Model file for the job. Use its own axes, mm. Face numbers are marked on the shaded views. A direction names the side the tool comes from. Round coordinates to 2 decimals unless told otherwise and drop trailing zeros. Loops run counter-clockwise (first coordinate to the right, second up) from the corner with the lowest first, then second, coordinate; pieces in that order, holes last. Notation, with made-up numbers: (48.5, 1.25) -> (100.5, 1.25) arc R5 cw to (100.5, 5.25) -> close; hole circle Ø10 at (22.5, -8.5). An arc over 180 degrees is marked (long way). Use a Markdown table: item, result.
from build123d import *

# Parameters (mm, degrees)
SKETCH2_R           = 0.6
BOSS_EXTRUDE2_DEPTH = 5
BOSS_EXTRUDE4_START = 15
BOSS_EXTRUDE4_DEPTH = 15
SKETCH8_R           = 1.5
CUT_EXTRUDE2_DEPTH  = 21.756494148


with BuildPart() as part:
    # Sketch2 → Boss-Extrude2 (new body)
    with BuildSketch(Plane.XY):
        with BuildLine():
            Line((-11.842719282, 4), (11.842719282, 4))
            Line((11.842719282, 4), (12.369316877, 4))
            ThreePointArc((12.369316877, 4), (13, 0), (12.369316877, -4))
            Line((12.369316877, -4), (11.842719282, -4))
            Line((11.842719282, -4), (-11.842719282, -4))
            Line((-11.842719282, -4), (-12.369316877, -4))
            ThreePointArc((-12.369316877, -4), (-13, 0), (-12.369316877, 4))
            Line((-12.369316877, 4), (-11.842719282, 4))
        make_face()
        with Locations((10, 0)):
            Circle(SKETCH2_R, mode=Mode.SUBTRACT)
        with Locations(Location((-10, 0, 0), (0, 0, 180))):
            Circle(SKETCH2_R, mode=Mode.SUBTRACT)
    extrude(amount=BOSS_EXTRUDE2_DEPTH)

    # Sketch7 → Boss-Extrude4 (add)
    with BuildSketch(Plane(origin=(0, 0, 0), x_dir=(-1, 0, 0), z_dir=(0, 0, -1)).offset(BOSS_EXTRUDE4_START)):
        with BuildLine():
            Line((0, -2.068941366), (-12.32759026, -2.068941366))
            Line((-12.32759026, -2.068941366), (-12.834308771, -2.068941366))
            ThreePointArc((-12.834308771, -2.068941366), (-12.6387473, -3.04336437), (-12.369316877, -4))
            Line((-12.369316877, -4), (-11.842719282, -4))
            Line((-11.842719282, -4), (0, -4))
            Line((0, -4), (11.842719282, -4))
            Line((11.842719282, -4), (12.369316877, -4))
            ThreePointArc((12.369316877, -4), (12.6387473, -3.04336437), (12.834308771, -2.068941366))
            Line((12.834308771, -2.068941366), (12.32759026, -2.068941366))
            Line((12.32759026, -2.068941366), (0, -2.068941366))
        make_face()
    extrude(amount=-BOSS_EXTRUDE4_DEPTH)

    # Sketch8 → Cut-Extrude2 (cut, through all)
    with BuildSketch(Plane(origin=(0, -2.068941366, 0), x_dir=(1, 0, 0), z_dir=(0, 1, 0))):
        with Locations(Location((-10.795, 7.5, 0), (0, 0, 270))):
            Circle(SKETCH8_R)
        with Locations(Location((10.795, 7.5, 0), (0, 0, 90))):
            Circle(SKETCH8_R)
    extrude(amount=-CUT_EXTRUDE2_DEPTH, mode=Mode.SUBTRACT)


solid = part.part
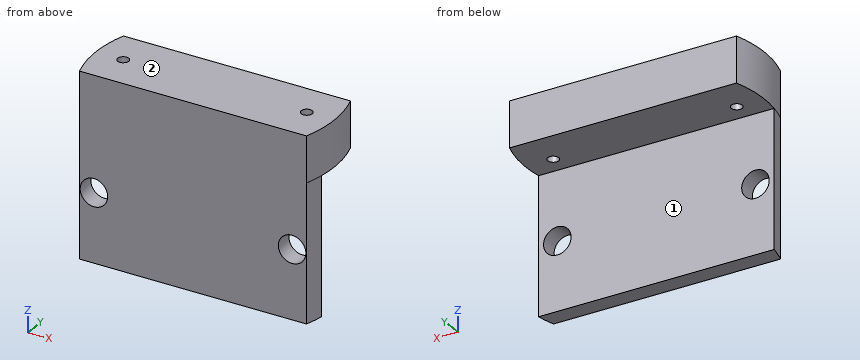
Q1. Flat gauge pins, fed straight in: pin 1 (10 mm diameter, centred on x = 8.5, z = -8, fed in from +Y); pin 2 (0.7 mm diameter, centred on x = 10, y = 0, fed in from +Z); pin 3 (1.9 mm diameter, centred on x = -10, y = 0, fed in from -Z). Where does each tip first touch, or does it go through?
Results list:
| item | result |
|---|---|
| pin 1 | stops at y = -2.07 |
| pin 2 | passes through |
| pin 3 | stops at z = 0 |
Q2. Band-saw the part on A-A, the plane z = -7.5. Give the cut face in (x, y) (3 decimals), plus the area to 3 significant figures.
Results list:
| item | result |
|---|---|
| outline | (-12.834, -2.069) arc R13 ccw to (-12.369, -4) -> (-12.295, -4) -> (-12.295, -2.069) -> close; (-9.295, -4) -> (9.295, -4) -> (9.295, -2.069) -> (-9.295, -2.069) -> close; (12.295, -4) -> (12.369, -4) arc R13 ccw to (12.834, -2.069) -> (12.295, -2.069) -> close |
| area | 37.2 mm² |
Q3. Drill centre lines: L1, parallel to Y at x = 10, z = 1.55; L2, parallel to X at y = -2.5, z = -7.5 (3 decimals); L3, parallel to X at y = -2.5, z = -8.75. Where is each one in solid material? Low to high. Write a range as from..to.
Results list:
| item | result |
|---|---|
| L1 | y = -4..-0.6, 0.6..4 |
| L2 | x = -12.757..-12.295, -9.295..9.295, 12.295..12.757 |
| L3 | x = -12.76..-11.62, -9.97..9.97, 11.62..12.76 |
Q4. Band-saw the part on D-D, the plane x = -6. Give the cut face in (y, z), plus the area to 3 significant figures.
Results list:
| item | result |
|---|---|
| outline | (-4, -15) -> (-2.07, -15) -> (-2.07, 0) -> (4, 0) -> (4, 5) -> (-4, 5) -> close |
| area | 69.0 mm² |
Q5. Tool access for the marked faces 1 and 2: list every direction of +Z, -Z, +X, -X, +Y, -Y with a clear straight run to the whole face (end or side of a thin tool).
Results list:
| item | result |
|---|---|
| face 1 | -Z, +X, -X, +Y |
| face 2 | +Z, +X, -X, +Y, -Y |
Q6. Band-saw the part on B-B, the plane y = 0. Give the cut face in (x, z), plus the area to 3 significant figures.
Results list:
| item | result |
|---|---|
| outline | (-13, 0) -> (-10.6, 0) -> (-10.6, 5) -> (-13, 5) -> close; (-9.4, 0) -> (9.4, 0) -> (9.4, 5) -> (-9.4, 5) -> close; (10.6, 0) -> (13, 0) -> (13, 5) -> (10.6, 5) -> close |
| area | 118 mm² |
Q7. Band-saw the part on C-C, the plane x = -10. Give the cut face in (y, z), plus the area to 3 significant figures.
Results list:
| item | result |
|---|---|
| outline | (-4, -15) -> (-2.07, -15) -> (-2.07, -8.77) -> (-4, -8.77) -> close; (-4, -6.23) -> (-2.07, -6.23) -> (-2.07, 0) -> (-0.6, 0) -> (-0.6, 5) -> (-4, 5) -> close; (0.6, 0) -> (4, 0) -> (4, 5) -> (0.6, 5) -> close |
| area | 58.1 mm² |
